The drawing under review shows one solid part. Ordinate dimensions are in mm from its lowest x, y, z. A direction names the side the tool comes from. Give positions to 0.01 mm unless a question says otherwise; leave off trailing zeros. Order: outer loops, then holes, each group sorted by start corner. A loop starts at its lowest first (then second) coordinate and runs counter-clockwise, first axis right, second up. Notation, with made-up numbers: (7, 53) -> (37, 53) arc R21 cw to (37, 74) -> close; hole circle Ø7 at (40, 41.25). An arc over 180 degrees is marked (long way). One line per item, written item: value. Start each with the question number.
1) Consider section B-B (z = 5.5). State the section outline as (x, y) points, plus the area to 3 significant figures.
2) Wall thickness on line 1 along Z through (x, y) = (3.75, 13.5); line 2 along Y through (x, z) = (1.75, 52); line 3 along Z through (x, y) = (1, 43): over which ranges is each line inside the solid? List them lowest first. Write a range as from..to.
3) Consider section D-D (z = 62). State the section outline as (x, y) points.
4) For pin 1 (2 mm diameter, centred on x = 4.5, z = 19, fed in from -Y); pin 2 (12 mm diameter, centred on y = 60.5, z = 18, fed in from -X), all flat-tipped, find the tip position at first contact; note any pin that passes through.
5) Consider section C-C (y = 20). State the section outline as (x, z) points, plus the area to 3 significant figures.
6) Consider section A-A (x = 4). State the section outline as (y, z) points.
7) Tool access review of the marked faces 1 and 2: name each direction out of +Z, -Z, +X, -X, +Y, -Y from which nothing blocks a thin tool from reaching the whole face with its end or side.
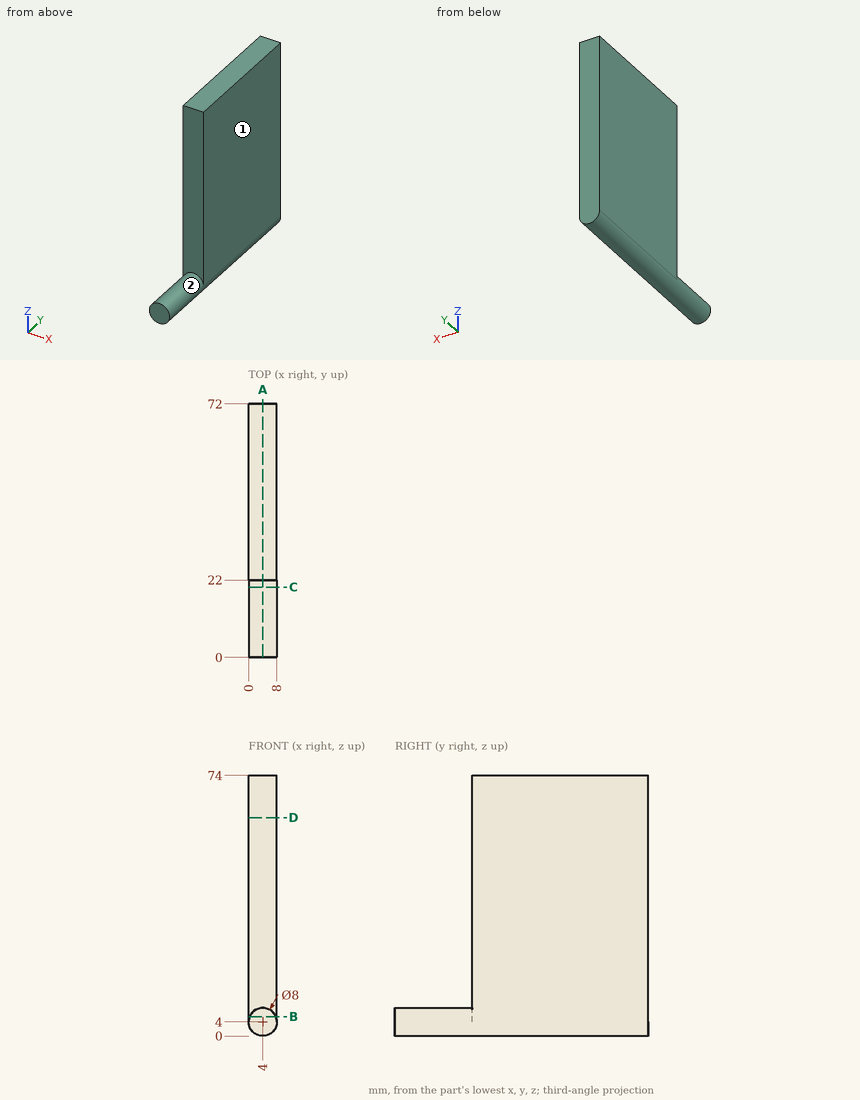
Checked values:
1. outline: (0, 22) -> (0.29, 22) -> (0.29, 0) -> (7.71, 0) -> (7.71, 22) -> (8, 22) -> (8, 72) -> (0, 72) -> close
1. area: 563 mm^2
2. line 1: z = 0.01..7.99
2. line 2: y = 22..72
2. line 3: z = 1.35..74
3. outline: (0, 22) -> (8, 22) -> (8, 72) -> (0, 72) -> close
4. pin 1: stops at y = 22
4. pin 2: stops at x = 0
5. outline: circle Ø8 at (4, 4)
5. area: 50.3 mm^2
6. outline: (0, 0) -> (72, 0) -> (72, 74) -> (22, 74) -> (22, 8) -> (0, 8) -> close
7. face 1: +Z, -Z, +X, +Y, -Y
7. face 2: -Y
